from build123d import *

# Parameters (mm, degrees)
F1_DEPTH = 50.8
F2_W     = 12.7
F2_H     = 12.7
F3_DEPTH = 25.4


with BuildPart() as f1:
    # F0 (on Front) → F1 (new body)
    with BuildSketch(Plane.XZ):
        Polygon((0, 50.79394), (-50.015371, 50.021338), (-50.015371, 0), (0.784629, 0), align=None)
    extrude(amount=F1_DEPTH)

    # F2 (on face) → F3 (join)
    with BuildSketch(Plane.XZ.offset(50.8)):
        with Locations((-43.665371, 6.35)):
            Rectangle(F2_W, F2_H)
    extrude(amount=F3_DEPTH)


solid = f1.part
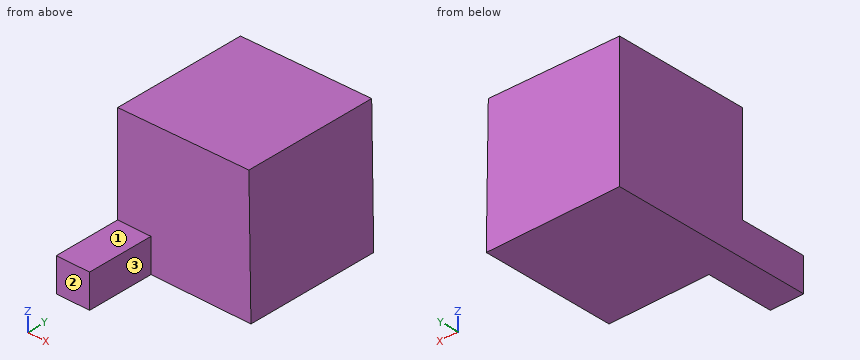
Design review of the part built by this model. Coordinates are the model's own, in mm. Face numbers are marked on the shaded views. A direction names the side the tool comes from. Round coordinates to 2 decimals unless told otherwise and drop trailing zeros. Write each loop counter-clockwise with the first axis right and the second up, starting at its lowest first coordinate (ties: lowest second). Pieces come first, ordered by that corner, then holes. Notation, with made-up numbers: (24, 33) - (46, 33) arc R27 ccw to (46, 72) - close; hole circle Ø7 at (69, 38). An arc over 180 degrees is marked (long way). Use a Markdown table: item, result. Add a question column.
1. Wall thickness on probe 1 along Y at (x, z) = (-33, 4.5); probe 2 along Z at (x, y) = (-46.5, -70); probe 3 along X at (y, z) = (-59.5, 9): over which ranges is each line inside the solid? List them lowest first.
2. We need section B-B (z = 7.5). State the section outline as (x, y) points, then the cut area to 3 significant figures.
3. We need section A-A (y = -30). State the section outline as (x, z) points.
4. We need section C-C (x = -8). State the section outline as (y, z) points, then the cut area to 3 significant figures.
5. For the marked faces 1, 2 and 3, list the 3-axis set-ups (+Z, -Z, +X, -X, +Y, -Y) from which the entire face can be reached by the end or side of a thin tool; tool diameter is ignored.
6. Clearance check with flat-ended pins moving along their axes: pin 1 (14 mm diameter, centred on x = -43, y = -65, fed in from +Z); pin 2 (4 mm diameter, centred on y = -57.5, z = 6.5, fed in from +X); pin 3 (8 mm diameter, centred on x = -40.5, z = 31, fed in from -Y). State where each tip first meets the part, or that it passes through.
Output:
| question | item | result |
|---|---|---|
| 1 | probe 1 | y = -50.8 to 0 |
| 1 | probe 2 | z = 0 to 12.7 |
| 1 | probe 3 | x = -50.02 to -37.32 |
| 2 | outline | (-50.02, -76.2) - (-37.32, -76.2) - (-37.32, -50.8) - (0.67, -50.8) - (0.67, 0) - (-50.02, 0) - close |
| 2 | area | 2,900 mm2 |
| 3 | outline | (-50.02, 0) - (0.78, 0) - (0, 50.79) - (-50.02, 50.02) - close |
| 4 | outline | (-50.8, 0) - (0, 0) - (0, 50.67) - (-50.8, 50.67) - close |
| 4 | area | 2,570 mm2 |
| 5 | face 1 | +Z, +X, -X, -Y |
| 5 | face 2 | +Z, -Z, +X, -X, -Y |
| 5 | face 3 | +Z, -Z, +X, -Y |
| 6 | pin 1 | stops at z = 12.7 |
| 6 | pin 2 | stops at x = -37.32 |
| 6 | pin 3 | stops at y = -50.8 |
